Verification items for the finished model (mm, model axes). Face numbers are marked on the shaded views. A direction names the side the tool comes from. Round coordinates to 2 decimals unless told otherwise and drop trailing zeros. Write each loop counter-clockwise with the first axis right and the second up, starting at its lowest first coordinate (ties: lowest second). Pieces come first, ordered by that corner, then holes. Notation, with made-up numbers: (-4.75, 50.5) - (49.25, 50.5) arc R23 ccw to (49.25, 86.5) - close; hole circle Ø3 at (10.25, 63.5). An arc over 180 degrees is marked (long way). Answer as a JSON object with one key per item and string values.
```python
from build123d import *

# Parameters (mm, degrees)
ESQUISSE1_W             = 254
ESQUISSE1_H             = 70
BOSS_EXTRU_1_DEPTH      = 5
ESQUISSE2_R             = 12.5
ENL_V_MAT_EXTRU_1_DEPTH = 132.829435256
BOSS_EXTRU_2_START      = 10
ESQUISSE3_R             = 17.5
ESQUISSE3_R_2           = 12.5
BOSS_EXTRU_2_DEPTH      = 10
ENL_V_MAT_EXTRU_2_DEPTH = 133.113587492
ESQUISSE5_W             = 45
ESQUISSE5_H             = 70
BOSS_EXTRU_3_DEPTH      = 4
ESQUISSE6_W             = 45
ESQUISSE6_H             = 70
BOSS_EXTRU_4_DEPTH      = 4
ESQUISSE7_R             = 2.5
ENL_V_MAT_EXTRU_3_DEPTH = 268.336866145
BOSS_EXTRU_5_START      = -4
ESQUISSE8_R             = 12.5
ESQUISSE8_R_2           = 8.5
BOSS_EXTRU_5_DEPTH      = 4


with BuildPart() as part:
    # Esquisse1 → Boss.-Extru.1 (new body)
    with BuildSketch(Plane.XY):
        Rectangle(ESQUISSE1_W, ESQUISSE1_H)
    extrude(amount=BOSS_EXTRU_1_DEPTH)

    # Esquisse2 → Enlèv. mat.-Extru.1 (cut, through all)
    with BuildSketch(Plane.XY.offset(5)):
        Circle(ESQUISSE2_R)
    extrude(amount=-ENL_V_MAT_EXTRU_1_DEPTH, mode=Mode.SUBTRACT)

    # Esquisse3 → Boss.-Extru.2 (add)
    with BuildSketch(Plane.XY.offset(5).offset(BOSS_EXTRU_2_START)):
        Circle(ESQUISSE3_R)
        Circle(ESQUISSE3_R_2, mode=Mode.SUBTRACT)
    extrude(amount=-BOSS_EXTRU_2_DEPTH)

    # Esquisse4 → Enlèv. mat.-Extru.2 (cut, through all)
    with BuildSketch(Plane.XY.offset(5)):
        with BuildLine():
            Line((-100, 12), (-40, 12))
            ThreePointArc((-40, 12), (-28, 0), (-40, -12))
            Line((-40, -12), (-100, -12))
            ThreePointArc((-100, -12), (-112, 0), (-100, 12))
        make_face()
        with BuildLine():
            Line((100, 12), (40, 12))
            ThreePointArc((40, 12), (28, 0), (40, -12))
            Line((40, -12), (100, -12))
            ThreePointArc((100, -12), (112, 0), (100, 12))
        make_face()
    extrude(amount=-ENL_V_MAT_EXTRU_2_DEPTH, mode=Mode.SUBTRACT)

    # Esquisse5 → Boss.-Extru.3 (add)
    with BuildSketch(Plane.ZY.offset(127)):
        with Locations((-17.5, 0)):
            Rectangle(ESQUISSE5_W, ESQUISSE5_H)
    extrude(amount=BOSS_EXTRU_3_DEPTH)

    # Esquisse6 → Boss.-Extru.4 (add)
    with BuildSketch(Plane(origin=(127, 0, 0), x_dir=(0, 0, -1), z_dir=(1, 0, 0))):
        with Locations((17.5, 0)):
            Rectangle(ESQUISSE6_W, ESQUISSE6_H)
    extrude(amount=BOSS_EXTRU_4_DEPTH)

    # Esquisse7 → Enlèv. mat.-Extru.3 (cut, through all)
    with BuildSketch(Plane.ZY.offset(131)):
        with Locations((-11, 30)):
            Circle(ESQUISSE7_R)
        with Locations((-11, -30)):
            Circle(ESQUISSE7_R)
        with Locations((-30, 30)):
            Circle(ESQUISSE7_R)
        with Locations((-30, -30)):
            Circle(ESQUISSE7_R)
    extrude(amount=-ENL_V_MAT_EXTRU_3_DEPTH, mode=Mode.SUBTRACT)

    # Esquisse8 → Boss.-Extru.5 (add)
    with BuildSketch(Plane(origin=(0, 0, 0), x_dir=(-1, 0, 0), z_dir=(0, 0, -1)).offset(BOSS_EXTRU_5_START)):
        with Locations(Location((0, 0, 0), (0, 0, 180))):
            Circle(ESQUISSE8_R)
        Circle(ESQUISSE8_R_2, mode=Mode.SUBTRACT)
    extrude(amount=BOSS_EXTRU_5_DEPTH)


solid = part.part
```
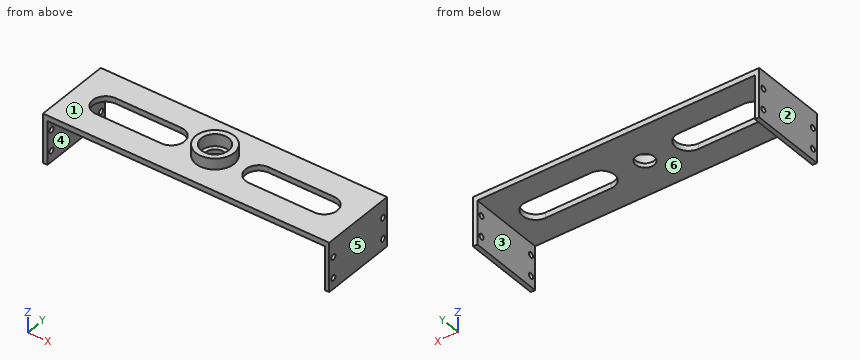
Q1. Gauge pin test, flat ends, axial feed: P1, Ø4.5, axis at y = -30, z = -11, coming from the -X side; P2, Ø5, axis at x = -54.5, y = -15.5, coming from the +Z side. Record the tip position at first contact, or that the pin passes through.
Geometry check:
{"P1": "passes through", "P2": "stops at z = 5"}
Q2. Section check C-C, the plane z = -11. Record the cut outline in (x, y), then the cut area to 3 significant figures.
Geometry check:
{"outline": "(-131, -35) - (-127, -35) - (-127, -32.5) - (-131, -32.5) - close; (-131, -27.5) - (-127, -27.5) - (-127, 27.5) - (-131, 27.5) - close; (-131, 32.5) - (-127, 32.5) - (-127, 35) - (-131, 35) - close; (127, -35) - (131, -35) - (131, -32.5) - (127, -32.5) - close; (127, -27.5) - (131, -27.5) - (131, 27.5) - (127, 27.5) - close; (127, 32.5) - (131, 32.5) - (131, 35) - (127, 35) - close", "area": "480 mm2"}
Q3. Material ranges on line 1 along Y through (x, z) = (128, -11); line 2 along X through (y, z) = (-8, -17); line 3 along Z through (x, y) = (37.5, 21.5), recorded low to high. Write a range as [from, to].
Geometry check:
{"line 1": "y = [-35, -32.5], [-27.5, 27.5], [32.5, 35]", "line 2": "x = [-131, -127], [127, 131]", "line 3": "z = [0, 5]"}
Q4. Section check D-D, the plane y = 0. Record the cut outline in (x, z).
Geometry check:
{"outline": "(-131, -40) - (-127, -40) - (-127, 0) - (-112, 0) - (-112, 5) - (-131, 5) - close; (-28, 0) - (-8.5, 0) - (-8.5, 4) - (-12.5, 4) - (-12.5, 15) - (-17.5, 15) - (-17.5, 5) - (-28, 5) - close; (8.5, 0) - (28, 0) - (28, 5) - (17.5, 5) - (17.5, 15) - (12.5, 15) - (12.5, 4) - (8.5, 4) - close; (112, 0) - (127, 0) - (127, -40) - (131, -40) - (131, 5) - (112, 5) - close"}
Q5. Section check A-A, the plane y = -30. Record the cut outline in (x, z).
Geometry check:
{"outline": "(-131, -40) - (-127, -40) - (-127, -32.5) - (-131, -32.5) - close; (-131, -27.5) - (-127, -27.5) - (-127, -13.5) - (-131, -13.5) - close; (-131, -8.5) - (-127, -8.5) - (-127, 0) - (127, 0) - (127, -8.5) - (131, -8.5) - (131, 5) - (-131, 5) - close; (127, -40) - (131, -40) - (131, -32.5) - (127, -32.5) - close; (127, -27.5) - (131, -27.5) - (131, -13.5) - (127, -13.5) - close"}
Q6. Set-up check for the marked faces 5 and 6: record each of +Z, -Z, +X, -X, +Y, -Y from which the full face is reachable in a straight line by a thin tool's end or side.
Geometry check:
{"face 5": "+Z, -Z, +X, +Y, -Y", "face 6": "-Z, +Y, -Y"}
Q7. Section check B-B, the plane x = 79.5. Record the cut outline in (y, z), then the cut area to 3 significant figures.
Geometry check:
{"outline": "(-35, 0) - (-12, 0) - (-12, 5) - (-35, 5) - close; (12, 0) - (35, 0) - (35, 5) - (12, 5) - close", "area": "230 mm2"}
Q8. Release check for a two-part mould opening along X. For the marked faces 1, 2, 3 and 4 record: released by +X, released by -X, zero draft, split by the parting line, or undercut.
Geometry check:
{"face 1": "zero draft", "face 2": "released by -X", "face 3": "undercut", "face 4": "undercut"}
